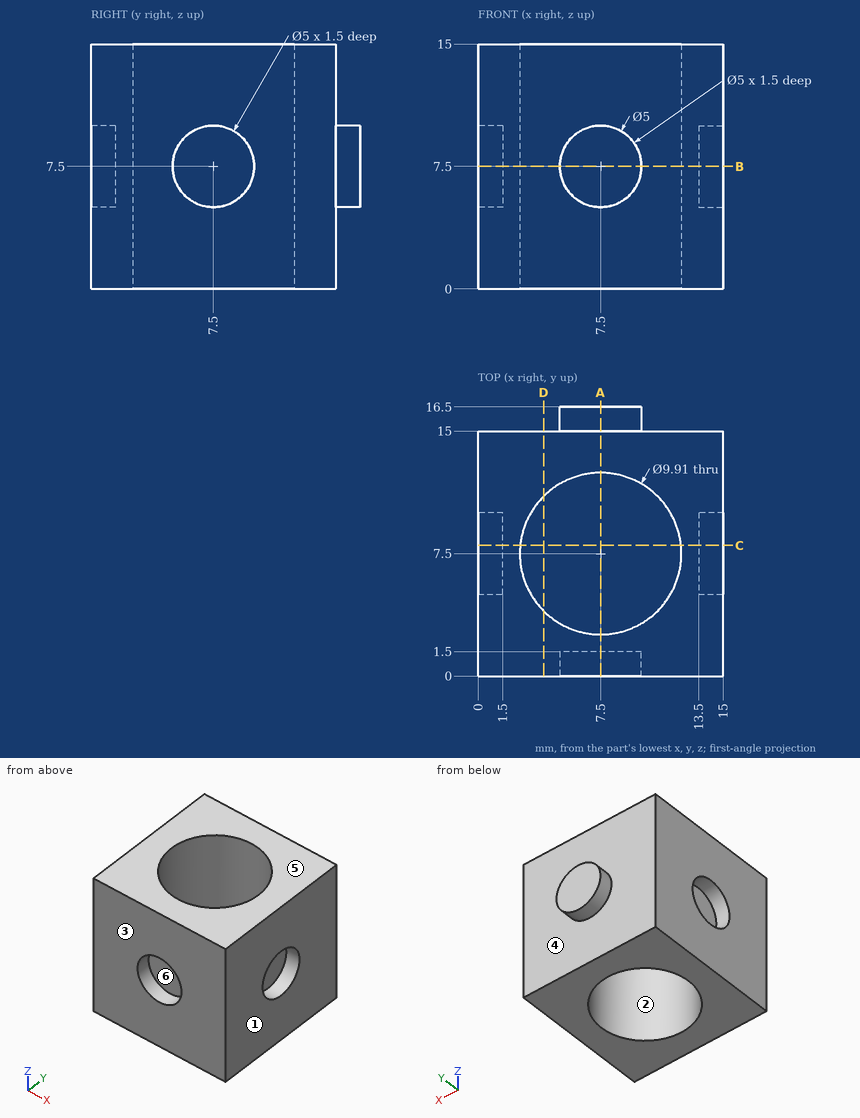
Source: three-view drawing plus pictorial views. Frame: mm from the lowest corner of the part. A direction names the side the tool comes from. Give positions to 0.01 mm unless a question says otherwise; leave off trailing zeros. Order: outer loops, then holes, each group sorted by start corner. A loop starts at its lowest first (then second) coordinate and runs counter-clockwise, first axis right, second up. Notation, with made-up numbers: (-1.75, 13.5) -> (32.25, 13.5) arc R28 ccw to (32.25, 45.5) -> close; hole circle Ø8 at (-1.5, -17.5). An arc over 180 degrees is marked (long way). Put each result on its own line as item: value.
Q1. Section B-B, the plane z = 7.5. Return loops of the section in (x, y) (3 decimals), then the cut area to 3 significant figures.
Here are the results:
outline: (0, 0) -> (5, 0) -> (5, 1.5) -> (10, 1.5) -> (10, 0) -> (15, 0) -> (15, 5) -> (13.5, 5) -> (13.5, 10) -> (15, 10) -> (15, 15) -> (10, 15) -> (10, 16.5) -> (5, 16.5) -> (5, 15) -> (0, 15) -> (0, 10) -> (1.5, 10) -> (1.5, 5) -> (0, 5) -> close; hole circle Ø9.91 at (7.5, 7.5)
area: 133 mm^2
Q2. Section C-C, the plane y = 8. Return loops of the section in (x, z), then the cut area to 3 significant figures.
Here are the results:
outline: (0, 0) -> (2.57, 0) -> (2.57, 15) -> (0, 15) -> (0, 9.95) -> (1.5, 9.95) -> (1.5, 5.05) -> (0, 5.05) -> close; (12.43, 0) -> (15, 0) -> (15, 5.05) -> (13.5, 5.05) -> (13.5, 9.95) -> (15, 9.95) -> (15, 15) -> (12.43, 15) -> close
area: 62.4 mm^2
Q3. Reachability of the marked faces 4, 5 and 6 from +Z, -Z, +X, -X, +Y, -Y: full face, straight path, thin tool, end or side. Return the list, or none.
Here are the results:
face 4: +Y
face 5: +Z, +X, -X, +Y, -Y
face 6: -Y
Q4. Material intervals for L1, parallel to Y at x = 1, z = 11.25; L2, parallel to Z at x = 0.65, y = 7.5; L3, parallel to X at y = 9, z = 12.75, sorted ascending.
Here are the results:
L1: y = 0 to 15
L2: z = 0 to 5, 10 to 15
L3: x = 0 to 2.78, 12.22 to 15
Q5. Section A-A, the plane x = 7.5. Return loops of the section in (y, z) (3 decimals).
Here are the results:
outline: (0, 0) -> (2.545, 0) -> (2.545, 15) -> (0, 15) -> (0, 10) -> (1.5, 10) -> (1.5, 5) -> (0, 5) -> close; (12.455, 0) -> (15, 0) -> (15, 5) -> (16.5, 5) -> (16.5, 10) -> (15, 10) -> (15, 15) -> (12.455, 15) -> close
Q6. Section D-D, the plane x = 4. Return loops of the section in (y, z).
Here are the results:
outline: (0, 0) -> (3.99, 0) -> (3.99, 15) -> (0, 15) -> close; (11.01, 0) -> (15, 0) -> (15, 15) -> (11.01, 15) -> close
Q7. Draft query along Y for the marked faces 1, 2 and 3. Return one class per face: released by +Y, released by -Y, zero draft, split by the parting line, or undercut.
Here are the results:
face 1: zero draft
face 2: undercut
face 3: released by -Y
Q8. Pin query (flat end, axial travel): pin 1 (4 mm diameter, centred on y = 7.5, z = 7.5, fed in from -X); pin 2 (2.5 mm diameter, centred on x = 8.5, z = 7, fed in from -Y); pin 3 (4.5 mm diameter, centred on y = 7.5, z = 7.5, fed in from +X). Return the tip coordinate at first contact, or that it passes through.
Here are the results:
pin 1: stops at x = 1.5
pin 2: stops at y = 1.5
pin 3: stops at x = 13.5
